Read the model definition and answer for the solid it produces. Units are mm, in the model's axes. Face numbers are marked on the shaded views. A direction names the side the tool comes from. Give positions to 0.01 mm unless a question says otherwise; leave off trailing zeros. Order: outer loops, then holes, each group sorted by start corner. A loop starts at its lowest first (then second) coordinate and runs counter-clockwise, first axis right, second up. Notation, with made-up numbers: (-15.5, -34) -> (40.5, -34) arc R23 cw to (40.5, -2) -> close; hole circle Ø10 at (-30, 71). An arc over 180 degrees is marked (long way). Use one line per item in the form item = value.
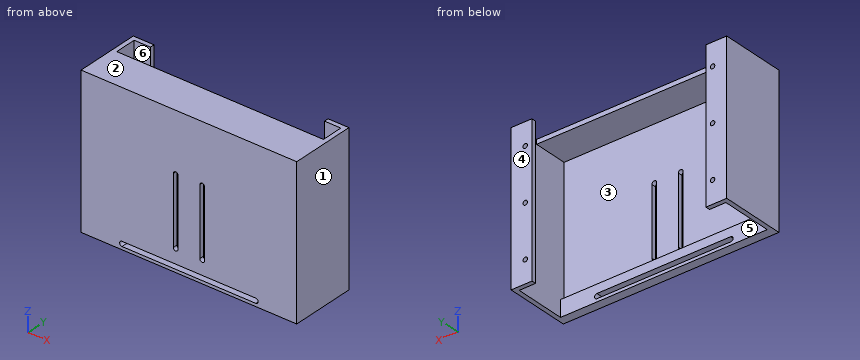
```python
from build123d import *

# Parameters (mm, degrees)
SKETCH_1_W          = 145
SKETCH_1_H          = 100
EXTRUDE_1_DEPTH     = 3
EXTRUDE_START       = 3
SKETCH_2_W          = 3
SKETCH_2_H          = 100
EXTRUDE_2_DEPTH     = 40.5
SKETCH_3_W          = 139
SKETCH_3_H          = 3
EXTRUDE_3_DEPTH     = 23
SKETCH_4_W          = 14
SKETCH_4_H          = 100
EXTRUDE_4_DEPTH     = 3
CUT_EXTRUDE_1_REACH = 100.227
SKETCH_5_R          = 1.5
CUT_EXTRUDE_2_REACH = 100.227
EXTRUDE_5_REACH     = 158.704
SKETCH_7_W          = 11
SKETCH_7_H          = 3
CUT_EXTRUDE_3_REACH = 97.721


with BuildPart() as part:
    # 草图1 → 凸台-拉伸1 (new body)
    with BuildSketch(Plane(origin=(0, 0, 0), x_dir=(1, 0, 0), z_dir=(0, 1, 0))):
        Rectangle(SKETCH_1_W, SKETCH_1_H)
    extrude(amount=EXTRUDE_1_DEPTH)

    # 草图2 → 凸台-拉伸2 (add)
    with BuildSketch(Plane(origin=(0, 0, 0), x_dir=(1, 0, 0), z_dir=(0, 1, 0)).offset(EXTRUDE_START)):
        with Locations((-71, 0)):
            Rectangle(SKETCH_2_W, SKETCH_2_H)
        with Locations((71, 0)):
            Rectangle(SKETCH_2_W, SKETCH_2_H)
    extrude(amount=EXTRUDE_2_DEPTH)

    # 草图3 → 凸台-拉伸3 (add)
    with BuildSketch(Plane(origin=(0, 3, 0), x_dir=(1, 0, 0), z_dir=(0, 1, 0))):
        with Locations((0, -48.5)):
            Rectangle(SKETCH_3_W, SKETCH_3_H)
    extrude(amount=EXTRUDE_3_DEPTH)

    # 草图4 → 凸台-拉伸4 (add)
    with BuildSketch(Plane(origin=(0, 43.5, 0), x_dir=(1, 0, 0), z_dir=(0, 1, 0))):
        with Locations((-65.5, 0)):
            Rectangle(SKETCH_4_W, SKETCH_4_H)
        with Locations((65.5, 0)):
            Rectangle(SKETCH_4_W, SKETCH_4_H)
    extrude(amount=-EXTRUDE_4_DEPTH)

    # 草图5 → 切除-拉伸1 (cut, up to next)
    with BuildSketch(Plane(origin=(0, 43.5, 0), x_dir=(1, 0, 0), z_dir=(0, 1, 0)), mode=Mode.PRIVATE) as cut_extrude_1_sk1:
        with Locations(Location((-63, 35, 0), (0, 0, 270))):
            Circle(SKETCH_5_R)
    cut_extrude_1_tool1 = extrude(cut_extrude_1_sk1.sketch, amount=-CUT_EXTRUDE_1_REACH, mode=Mode.PRIVATE) & part.part
    # 草图5 → 切除-拉伸1 (cut, up to next)
    with BuildSketch(Plane(origin=(0, 43.5, 0), x_dir=(1, 0, 0), z_dir=(0, 1, 0)), mode=Mode.PRIVATE) as cut_extrude_1_sk2:
        with Locations(Location((-63, 0, 0), (0, 0, 270))):
            Circle(SKETCH_5_R)
    cut_extrude_1_tool2 = extrude(cut_extrude_1_sk2.sketch, amount=-CUT_EXTRUDE_1_REACH, mode=Mode.PRIVATE) & part.part
    # 草图5 → 切除-拉伸1 (cut, up to next)
    with BuildSketch(Plane(origin=(0, 43.5, 0), x_dir=(1, 0, 0), z_dir=(0, 1, 0)), mode=Mode.PRIVATE) as cut_extrude_1_sk3:
        with Locations(Location((-63, -35, 0), (0, 0, 270))):
            Circle(SKETCH_5_R)
    cut_extrude_1_tool3 = extrude(cut_extrude_1_sk3.sketch, amount=-CUT_EXTRUDE_1_REACH, mode=Mode.PRIVATE) & part.part
    # 草图5 → 切除-拉伸1 (cut, up to next)
    with BuildSketch(Plane(origin=(0, 43.5, 0), x_dir=(1, 0, 0), z_dir=(0, 1, 0)), mode=Mode.PRIVATE) as cut_extrude_1_sk4:
        with Locations(Location((63, -35, 0), (0, 0, 270))):
            Circle(SKETCH_5_R)
    cut_extrude_1_tool4 = extrude(cut_extrude_1_sk4.sketch, amount=-CUT_EXTRUDE_1_REACH, mode=Mode.PRIVATE) & part.part
    # 草图5 → 切除-拉伸1 (cut, up to next)
    with BuildSketch(Plane(origin=(0, 43.5, 0), x_dir=(1, 0, 0), z_dir=(0, 1, 0)), mode=Mode.PRIVATE) as cut_extrude_1_sk5:
        with Locations(Location((63, 0, 0), (0, 0, 270))):
            Circle(SKETCH_5_R)
    cut_extrude_1_tool5 = extrude(cut_extrude_1_sk5.sketch, amount=-CUT_EXTRUDE_1_REACH, mode=Mode.PRIVATE) & part.part
    # 草图5 → 切除-拉伸1 (cut, up to next)
    with BuildSketch(Plane(origin=(0, 43.5, 0), x_dir=(1, 0, 0), z_dir=(0, 1, 0)), mode=Mode.PRIVATE) as cut_extrude_1_sk6:
        with Locations(Location((63, 35, 0), (0, 0, 270))):
            Circle(SKETCH_5_R)
    cut_extrude_1_tool6 = extrude(cut_extrude_1_sk6.sketch, amount=-CUT_EXTRUDE_1_REACH, mode=Mode.PRIVATE) & part.part
    add(cut_extrude_1_tool1.solids().sort_by_distance((-63, 43.5, -35))[0], mode=Mode.SUBTRACT)
    add(cut_extrude_1_tool2.solids().sort_by_distance((-63, 43.5, 0))[0], mode=Mode.SUBTRACT)
    add(cut_extrude_1_tool3.solids().sort_by_distance((-63, 43.5, 35))[0], mode=Mode.SUBTRACT)
    add(cut_extrude_1_tool4.solids().sort_by_distance((63, 43.5, 35))[0], mode=Mode.SUBTRACT)
    add(cut_extrude_1_tool5.solids().sort_by_distance((63, 43.5, 0))[0], mode=Mode.SUBTRACT)
    add(cut_extrude_1_tool6.solids().sort_by_distance((63, 43.5, -35))[0], mode=Mode.SUBTRACT)

    # 草图6 → 切除-拉伸2 (cut, up to next)
    with BuildSketch(Plane.XZ, mode=Mode.PRIVATE) as cut_extrude_2_sk1:
        with BuildLine():
            Line((-7.3, 10.448254834), (-7.3, -35.117406069))
            ThreePointArc((-7.3, -35.117406069), (-8.9, -36.717406069), (-10.5, -35.117406069))
            Line((-10.5, -35.117406069), (-10.5, 10.448254834))
            ThreePointArc((-10.5, 10.448254834), (-8.9, 12.048254834), (-7.3, 10.448254834))
        make_face()
    cut_extrude_2_tool1 = extrude(cut_extrude_2_sk1.sketch, amount=-CUT_EXTRUDE_2_REACH, mode=Mode.PRIVATE) & part.part
    # 草图6 → 切除-拉伸2 (cut, up to next)
    with BuildSketch(Plane.XZ, mode=Mode.PRIVATE) as cut_extrude_2_sk2:
        with BuildLine():
            Line((7.3, 10.448254834), (7.3, -35.117406069))
            ThreePointArc((7.3, -35.117406069), (8.9, -36.717406069), (10.5, -35.117406069))
            Line((10.5, -35.117406069), (10.5, 10.448254834))
            ThreePointArc((10.5, 10.448254834), (8.9, 12.048254834), (7.3, 10.448254834))
        make_face()
    cut_extrude_2_tool2 = extrude(cut_extrude_2_sk2.sketch, amount=-CUT_EXTRUDE_2_REACH, mode=Mode.PRIVATE) & part.part
    add(cut_extrude_2_tool1.solids().sort_by_distance((-8.9, 0, -12.334576))[0], mode=Mode.SUBTRACT)
    add(cut_extrude_2_tool2.solids().sort_by_distance((8.9, 0, -12.334576))[0], mode=Mode.SUBTRACT)

    # 草图7 → 凸台-拉伸5 (add, up to next)
    with BuildSketch(Plane.ZY.offset(-69.5), mode=Mode.PRIVATE) as extrude_5_sk1:
        with Locations((-44.5, 4.5)):
            Rectangle(SKETCH_7_W, SKETCH_7_H)
    extrude_5_tool1 = extrude(extrude_5_sk1.sketch, amount=EXTRUDE_5_REACH, mode=Mode.PRIVATE) - part.part
    add(extrude_5_tool1.solids().sort_by_distance((69.5, 4.5, -44.5))[0])

    # 草图8 → 切除-拉伸3 (cut, up to next)
    with BuildSketch(Plane(origin=(0, 6, 0), x_dir=(1, 0, 0), z_dir=(0, 1, 0)), mode=Mode.PRIVATE) as cut_extrude_3_sk1:
        with BuildLine():
            Line((-45, 48), (45, 48))
            ThreePointArc((45, 48), (46.6, 46.4), (45, 44.8))
            Line((45, 44.8), (-45, 44.8))
            ThreePointArc((-45, 44.8), (-46.6, 46.4), (-45, 48))
        make_face()
    cut_extrude_3_tool1 = extrude(cut_extrude_3_sk1.sketch, amount=-CUT_EXTRUDE_3_REACH, mode=Mode.PRIVATE) & part.part
    add(cut_extrude_3_tool1.solids().sort_by_distance((0, 6, -46.4))[0], mode=Mode.SUBTRACT)


solid = part.part
```
Item 1: Given pin 1 Ø2.5 at (x, z) = (-29.5, 49) entering from +Y; pin 2 Ø2.5 at (x, z) = (63, 35) entering from +Y; pin 3 Ø7 at (x, y) = (-30, 12.5) entering from -Z, each flat-ended and moving along its own axis, determine where each tip first touches the part or whether it passes through.
Checks:
pin_1 = 26
pin_2 = 3
pin_3 = 47
Item 2: Which of the six approach directions +Z, -Z, +X, -X, +Y, -Y give full straight-line access (tool end or side, diameter ignored) to the marked faces 4, 5 and 6?
Checks:
face_4 = +Z, -Z, +X, -X, +Y
face_5 = -Z
face_6 = +Z, -Z
Item 3: Determine the mould class of the marked faces 1, 2 and 3 for opening direction Z: +Z half, -Z half, draft (parallel to the pull), parting line (faces both ways), or undercut.
Checks:
face_1 = draft
face_2 = +Z half
face_3 = undercut
Item 4: The part is cut by section B-B on z = -27. Give the vertices of the cut face in (x, y).
Checks:
outline = (-72.5, 0) -> (-10.5, 0) -> (-10.5, 3) -> (-69.5, 3) -> (-69.5, 40.5) -> (-58.5, 40.5) -> (-58.5, 43.5) -> (-72.5, 43.5) -> close; (-7.3, 0) -> (7.3, 0) -> (7.3, 3) -> (-7.3, 3) -> close; (10.5, 0) -> (72.5, 0) -> (72.5, 43.5) -> (58.5, 43.5) -> (58.5, 40.5) -> (69.5, 40.5) -> (69.5, 3) -> (10.5, 3) -> close
Item 5: The part is cut by section D-D on z = 0. Give the vertices of the cut face in (x, y).
Checks:
outline = (-72.5, 0) -> (-10.5, 0) -> (-10.5, 3) -> (-69.5, 3) -> (-69.5, 40.5) -> (-64.5, 40.5) -> (-64.5, 43.5) -> (-72.5, 43.5) -> close; (-61.5, 40.5) -> (-58.5, 40.5) -> (-58.5, 43.5) -> (-61.5, 43.5) -> close; (-7.3, 0) -> (7.3, 0) -> (7.3, 3) -> (-7.3, 3) -> close; (10.5, 0) -> (72.5, 0) -> (72.5, 43.5) -> (64.5, 43.5) -> (64.5, 40.5) -> (69.5, 40.5) -> (69.5, 3) -> (10.5, 3) -> close; (58.5, 40.5) -> (61.5, 40.5) -> (61.5, 43.5) -> (58.5, 43.5) -> close
Item 6: Straight lines are drawn through the part: L1, parallel to X at y = 42.15, z = 35; L2, parallel to Z at x = -57, y = 5; L3, parallel to X at y = 18, z = 34. For each, find the intervals that lie inside material, in ascending order. Write a range as from..to.
Checks:
L1 = -72.5..-64.5, -61.5..-58.5, 58.5..61.5, 64.5..72.5
L2 = -50..-39, 47..50
L3 = -72.5..-69.5, 69.5..72.5
Item 7: The part is cut by section A-A on x = 38. Give the vertices of the cut face in (y, z), and give its area (3 significant figures).
Checks:
outline = (0, -50) -> (6, -50) -> (6, -48) -> (0, -48) -> close; (0, -44.8) -> (6, -44.8) -> (6, -39) -> (3, -39) -> (3, 47) -> (26, 47) -> (26, 50) -> (0, 50) -> close
area = 383 mm²
Item 8: The part is cut by section C-C on y = 38.5. Give the vertices of the cut face in (x, z).
Checks:
outline = (-72.5, -50) -> (-69.5, -50) -> (-69.5, 50) -> (-72.5, 50) -> close; (69.5, -50) -> (72.5, -50) -> (72.5, 50) -> (69.5, 50) -> close
